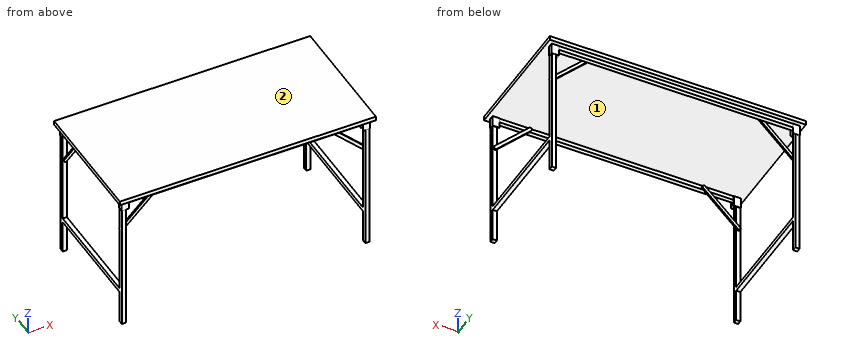
```python
from build123d import *

# Parameters (mm, degrees)
F0_W      = 1520
F0_H      = 750
F1_DEPTH  = 25
F2_W      = 1470
F2_H      = 25
F3_DEPTH  = 25
F5_DEPTH  = 65
F7_W      = 25
F7_H      = 25
F8_DEPTH  = 805
F10_DEPTH = 65
F12_W     = 25
F12_H     = 25
F13_DEPTH = 805
F15_W     = 25
F15_H     = 25
F16_DEPTH = 805
F18_W     = 25
F18_H     = 25
F19_DEPTH = 650
F21_W     = 25
F21_H     = 25
F22_DEPTH = 650
F24_DEPTH = 10
F26_DEPTH = 10
F29_DEPTH = 10
F31_DEPTH = 10


with BuildPart() as f1:
    # F0 (on Top) → F1 (new body)
    with BuildSketch(Plane.XY):
        with Locations((-760, 375)):
            Rectangle(F0_W, F0_H)
    extrude(amount=F1_DEPTH)

    # F2 (on face) → F3 (join)
    with BuildSketch(Plane(origin=(0, 0, 0), x_dir=(1, 0, 0), z_dir=(0, 0, -1))):
        with Locations((-760, -37.5)):
            Rectangle(F2_W, F2_H)
        with Locations((-760, -712.5)):
            Rectangle(F2_W, F2_H)
    extrude(amount=F3_DEPTH)

    # F4 (on face) → F5 (join)
    with BuildSketch(Plane(origin=(0, 0, 0), x_dir=(1, 0, 0), z_dir=(0, 0, -1))):
        Polygon((-65, -25), (-25, -25), (-25, -50), (-65, -50), (-65, -52), (-23, -52), (-23, -23), (-65, -23), align=None)
    extrude(amount=F5_DEPTH)

    # F7 (on offset) → F8 (join)
    with BuildSketch(Plane(origin=(0, 0, -35), x_dir=(1, 0, 0), z_dir=(0, 0, -1))):
        with Locations((-37.5, -37.523640207)):
            Rectangle(F7_W, F7_H)
    extrude(amount=F8_DEPTH)

    # F9 (on face) → F10 (join)
    with BuildSketch(Plane.XY):
        Polygon((-1495, 724.9829173088), (-1455, 724.9829173088), (-1455, 726.9829173088), (-1497, 726.9829173088), (-1497, 697.9829173088), (-1455, 697.9829173088), (-1455, 699.9829173088), (-1495, 699.9829173088), align=None)
        Polygon((-65.0490959734, 726.9829173088), (-65.0490959734, 724.9829173088), (-25.0490959734, 724.9829173088), (-25.0490959734, 699.9829173088), (-65.0490959734, 699.9829173088), (-65.0490959734, 697.9829173088), (-23.0490959734, 697.9829173088), (-23.0490959734, 726.9829173088), align=None)
        Polygon((-1455, 25), (-1495, 25), (-1495, 50), (-1455, 50), (-1455, 52), (-1497, 52), (-1497, 23), (-1455, 23), align=None)
    extrude(amount=-F10_DEPTH)

    # F12 (on offset) → F13 (join)
    with BuildSketch(Plane(origin=(0, 0, -35), x_dir=(1, 0, 0), z_dir=(0, 0, -1))):
        with Locations((-1482.5, -37.5)):
            Rectangle(F12_W, F12_H)
    extrude(amount=F13_DEPTH)

    # F15 (on offset) → F16 (join)
    with BuildSketch(Plane(origin=(0, 0, -35), x_dir=(1, 0, 0), z_dir=(0, 0, -1))):
        with Locations((-37.5, -712.5)):
            Rectangle(F15_W, F15_H)
        with Locations((-1482.5, -712.5)):
            Rectangle(F15_W, F15_H)
    extrude(amount=F16_DEPTH)

    # F18 (on offset) → F19 (join)
    with BuildSketch(Plane(origin=(0, 50.023640207, 0), x_dir=(-1, 0, 0), z_dir=(0, 1, 0))):
        with Locations((37.5, -627.5)):
            Rectangle(F18_W, F18_H)
    extrude(amount=F19_DEPTH)

    # F21 (on offset) → F22 (join)
    with BuildSketch(Plane(origin=(0, 50, 0), x_dir=(-1, 0, 0), z_dir=(0, 1, 0))):
        with Locations((1482.5, -627.5)):
            Rectangle(F21_W, F21_H)
    extrude(amount=F22_DEPTH)

    # F23 (on face) → F24 (join)
    with BuildSketch(Plane.XZ.offset(-700)):
        with BuildLine():
            Line((-50, -190.7444713597), (-234.6244849475, -9.2794851613))
            ThreePointArc((-234.6244849475, -9.2794851613), (-246.6039118675, -7.7336055545), (-251.332803081, -18.8481906111))
            Line((-251.332803081, -18.8481906111), (-50, -216.7355636904))
            Line((-50, -216.7355636904), (-50, -190.7444713597))
        make_face()
        with BuildLine():
            Line((-27.8014624786, -212.5631229112), (-50, -190.7444713597))
            Line((-50, -190.7444713597), (-50, -216.7355636904))
            Line((-50, -216.7355636904), (-44.5097806121, -222.131828361))
            ThreePointArc((-44.5097806121, -222.131828361), (-32.5303536921, -223.6777079678), (-27.8014624786, -212.5631229112))
        make_face()
    extrude(amount=F24_DEPTH)

    # F25 (on face) → F26 (join)
    with BuildSketch(Plane(origin=(0, 50.023640207, 0), x_dir=(-1, 0, 0), z_dir=(0, 1, 0))):
        with BuildLine():
            Line((50, -188.6229664357), (50, -216.7160920101))
            Line((50, -216.7160920101), (250.9788283543, -18.4630064225))
            ThreePointArc((250.9788283543, -18.4630064225), (251.07538107, -4.3212004002), (236.9335750477, -4.2246476845))
            Line((236.9335750477, -4.2246476845), (50, -188.6229664357))
        make_face()
        with BuildLine():
            ThreePointArc((30.4773733467, -207.880820631), (30.380820631, -222.0226266533), (44.5226266533, -222.119179369))
            Line((44.5226266533, -222.119179369), (50, -216.7160920101))
            Line((50, -216.7160920101), (50, -188.6229664357))
            Line((50, -188.6229664357), (30.4773733467, -207.880820631))
        make_face()
    extrude(amount=F26_DEPTH)

    # F28 (on offset) → F29 (join)
    with BuildSketch(Plane.XZ.offset(-700)):
        with BuildLine():
            ThreePointArc((-1268.519621658, -19.0091897955), (-1268.3869301053, -4.8676766886), (-1282.5284432121, -4.7349851358))
            Line((-1282.5284432121, -4.7349851358), (-1489.504410777, -207.8628976702))
            ThreePointArc((-1489.504410777, -207.8628976702), (-1489.6371023298, -222.004410777), (-1475.495589223, -222.1371023298))
            Line((-1475.495589223, -222.1371023298), (-1268.519621658, -19.0091897955))
        make_face()
    extrude(amount=F29_DEPTH)

    # F30 (on face) → F31 (join)
    with BuildSketch(Plane(origin=(0, 50, 0), x_dir=(-1, 0, 0), z_dir=(0, 1, 0))):
        with BuildLine():
            ThreePointArc((1475.506314972, -222.1476128693), (1489.6476128693, -221.993685028), (1489.493685028, -207.8523871307))
            Line((1489.493685028, -207.8523871307), (1470, -188.7785095141))
            Line((1470, -188.7785095141), (1470, -216.7598794703))
            Line((1470, -216.7598794703), (1475.506314972, -222.1476128693))
        make_face()
        with BuildLine():
            Line((1470, -216.7598794703), (1470, -188.7785095141))
            Line((1470, -188.7785095141), (1282.212911818, -5.0355213195))
            ThreePointArc((1282.212911818, -5.0355213195), (1268.0716139207, -5.1894491609), (1268.225541762, -19.3307470582))
            Line((1268.225541762, -19.3307470582), (1470, -216.7598794703))
        make_face()
    extrude(amount=F31_DEPTH)


solid = f1.part
```
Model file for the job. Use its own axes, mm. Face numbers are marked on the shaded views. Coordinates: 2 decimals unless noted, no trailing zeros. Loops run counter-clockwise (first coordinate to the right, second up) from the corner with the lowest first, then second, coordinate; pieces in that order, holes last. Notation, with made-up numbers: (-13.5, -39.5) - (1.5, -39.5) arc R16 cw to (1.5, -12.5) - close; hole circle Ø11 at (82.5, 18.25). An arc over 180 degrees is marked (long way). Write item = value, one per line. Start each with the question number.
Item 1: Saw through at D-D, the plane x = -587. List the corners of the cut face in (y, z), then the cut area to 3 significant figures.
Item 2: Saw through at B-B, the plane z = -422. List the corners of the cut face in (x, y).
Item 3: Pull direction Y, two halves, no side cores. Call the marked faces 1 and 2: +Y half, -Y half, draft (parallel to the pull), parting line (faces both ways), or undercut.
Item 4: Drop flat-ended pins along their axis: pin 1 Ø14.5 at (y, z) = (718.5, -47.5) entering from +X; pin 2 Ø0.6 at (y, z) = (24.5, -26.5) entering from -X; pin 3 Ø20 at (x, z) = (-654, -15.5) entering from -Y. Give the stop position or say it passes through.
Item 5: Saw through at A-A, the plane y = 122. List the corners of the cut face in (x, z).
Item 6: Wall check: probe 1 along X at (y, z) = (531, -637); probe 2 along Z at (x, y) = (-1138.5, 206.5); probe 3 along Y at (x, z) = (-668.5, -11). Give the ranges that are in metal, low to high. Write a range as [from, to].
Item 7: Saw through at C-C, the plane x = -1328.5. List the corners of the cut face in (y, z).
Answers:
q1.outline = (0, 0) - (25, 0) - (25, -25) - (50, -25) - (50, 0) - (700, 0) - (700, -25) - (725, -25) - (725, 0) - (750, 0) - (750, 25) - (0, 25) - close
q1.area = 20,000 mm2
q2.outline = (-1495, 25) - (-1470, 25) - (-1470, 50) - (-1495, 50) - close; (-1495, 700) - (-1470, 700) - (-1470, 725) - (-1495, 725) - close; (-50, 25.02) - (-25, 25.02) - (-25, 50.02) - (-50, 50.02) - close; (-50, 700) - (-25, 700) - (-25, 725) - (-50, 725) - close
q3.face_1 = undercut
q3.face_2 = draft
q4.pin_1 = -23.05
q4.pin_2 = -1497
q4.pin_3 = 25
q5.outline = (-1520, 0) - (0, 0) - (0, 25) - (-1520, 25) - close; (-1495, -640) - (-1470, -640) - (-1470, -615) - (-1495, -615) - close; (-50, -640) - (-25, -640) - (-25, -615) - (-50, -615) - close
q6.probe_1 = [-1495, -1470], [-50, -25]
q6.probe_2 = [0, 25]
q6.probe_3 = [25, 50], [700, 725]
q7.outline = (0, 0) - (25, 0) - (25, -25) - (50, -25) - (50, 0) - (700, 0) - (700, -25) - (725, -25) - (725, 0) - (750, 0) - (750, 25) - (0, 25) - close; (50, -78.31) - (60, -78.31) - (60, -50.33) - (50, -50.33) - close; (690, -77.87) - (700, -77.87) - (700, -49.85) - (690, -49.85) - close
